Check sheet for the modelled part. Datum: model origin and axes. Units: mm. A direction names the side the tool comes from. Round coordinates to 2 decimals unless told otherwise and drop trailing zeros. Order: outer loops, then holes, each group sorted by start corner. A loop starts at its lowest first (then second) coordinate and runs counter-clockwise, first axis right, second up.
Q1. Cross-section at C-C on z = 2.5. Record the cut outline in (x, y).
Q2. Cross-section at B-B on x = -10. Record the cut outline in (y, z).
Q3. Set-up check for faces 1 (the flat face through (1.905, -122, 20)), 2 (the flat face through (-10.63, -56.35, 6.13)), 3 (the flat face through (0, 5, 19.987)): record each of +Z, -Z, +X, -X, +Y, -Y from which the full face is reachable in a straight line by a thin tool's end or side.
Q4. Scan lines: probe 1 along Z at (x, y) = (-7, -46.5); probe 2 along Z at (x, y) = (-13, -58); probe 3 along Z at (x, y) = (5.5, -43). Record each from-to range of solid material in increasing order.
Q5. Cross-section at A-A on y = -32.5. Record the cut outline in (x, z).
Q6. Depth check by flat-ended pin: P1, Ø6, axis at x = -17.5, z = 14.5, coming from the +Y side; P2, Ø1.1, axis at x = 0.5, y = 6, coming from the +Z side; P3, Ø6, axis at x = -9, z = 11, coming from the -Y side. Enter the tip coordinate at first touch or a pass-through.
Q7. Mould release check, pull along Z, two halves, no side actions. Record for faces 4 (the flat face through (6.61, -56.35, 4.62)), 5 (the flat face through (-1.905, -122, 20)), 6 (the flat face through (0, 6, 23.797)), 7 (the cylindrical face through (17.27, -56.35, 10.71)): +Z half, -Z half, draft (parallel to the pull), parting line (faces both ways), or undercut.
from build123d import *

# Parameters (mm, degrees)
F0_R     = 25.4
F1_DEPTH = 114.3
F2_W     = 3.81
F2_H     = 3.81
F3_DEPTH = 12.7
F4_W     = 3.81
F4_H     = 3.81
F5_DEPTH = 12.7
F6_W     = 3.81
F6_H     = 3.556
F7_DEPTH = 6.35
F8_W     = 3.81
F8_H     = 3.556
F9_DEPTH = 6.35


with BuildPart() as f1:
    # F0 (on Front) → F1 (new body)
    with BuildSketch(Plane.XZ):
        Circle(F0_R)
        with BuildLine():
            ThreePointArc((16.884709, -11.305264), (0.394939, -20.316162), (-16.432577, -11.952941))
            Line((-16.432577, -11.952941), (16.884709, -11.305264))
        make_face(mode=Mode.SUBTRACT)
        with BuildLine():
            ThreePointArc((-18.567839, -8.254559), (-17.791782, 9.816053), (-2.919006, 20.109247))
            Line((-2.919006, 20.109247), (-18.567839, -8.254559))
        make_face(mode=Mode.SUBTRACT)
        Polygon((0.19747, 15.241919), (13.196979, -6.295993), (-11.955155, -6.784942), align=None, mode=Mode.SUBTRACT)
        with BuildLine():
            ThreePointArc((3.221185, 20.06306), (17.396842, 10.500108), (19.252822, -6.498558))
            Line((19.252822, -6.498558), (3.221185, 20.06306))
        make_face(mode=Mode.SUBTRACT)
    extrude(amount=F1_DEPTH)

    # F2 (on face) → F3 (join)
    with BuildSketch(Plane(origin=(0, 0, 0), x_dir=(-1, 0, 0), z_dir=(0, 1, 0))):
        with Locations((0, 21.892242)):
            Rectangle(F2_W, F2_H)
    extrude(amount=F3_DEPTH)

    # F4 (on face) → F5 (join)
    with BuildSketch(Plane.XZ.offset(114.3)):
        with Locations((0, 21.180816)):
            Rectangle(F4_W, F4_H)
    extrude(amount=F5_DEPTH)

    # F6 (on face) → F7 (join)
    with BuildSketch(Plane(origin=(0, 0, 19.987242), x_dir=(1, 0, 0), z_dir=(0, 0, -1))):
        with Locations((0, -10.922)):
            Rectangle(F6_W, F6_H)
    extrude(amount=F7_DEPTH)

    # F8 (on face) → F9 (join)
    with BuildSketch(Plane(origin=(0, 0, 19.275816), x_dir=(1, 0, 0), z_dir=(0, 0, -1))):
        with Locations((0, 125.222)):
            Rectangle(F8_W, F8_H)
    extrude(amount=F9_DEPTH)


solid = f1.part
Results found:
1. outline: (-25.28, -114.3) - (-20.17, -114.3) - (-20.17, 0) - (-25.28, 0) - close; (-12.63, -114.3) - (-6.83, -114.3) - (-6.83, 0) - (-12.63, 0) - close; (7.89, -114.3) - (13.82, -114.3) - (13.82, 0) - (7.89, 0) - close; (20.17, -114.3) - (25.28, -114.3) - (25.28, 0) - (20.17, 0) - close
2. outline: (-114.3, -23.35) - (0, -23.35) - (0, -17.69) - (-114.3, -17.69) - close; (-114.3, -11.83) - (0, -11.83) - (0, -6.75) - (-114.3, -6.75) - close; (-114.3, -3.24) - (0, -3.24) - (0, 7.27) - (-114.3, 7.27) - close; (-114.3, 17.69) - (0, 17.69) - (0, 23.35) - (-114.3, 23.35) - close
3. face 1: +Z, -Z, +X, -Y
3. face 2: +Y, -Y
3. face 3: -Z, +X, -X
4. probe 1: z = -24.42 to -19.08, -11.77 to -6.69, 2.2 to 12.71, 19.08 to 24.42
4. probe 2: z = -21.82 to -15.62, -11.89 to 1.84, 15.62 to 21.82
4. probe 3: z = -24.8 to -19.56, -11.53 to -6.45, 6.46 to 16.29, 19.56 to 24.8
5. outline: circle Ø50.8 at (0, 0); hole (-18.57, -8.25) - (-2.92, 20.11) arc R20.32 ccw to start; hole (-16.43, -11.95) arc R20.32 ccw to (16.88, -11.31) - close; hole (-11.96, -6.78) - (13.2, -6.3) - (0.2, 15.24) - close; hole (3.22, 20.06) - (19.25, -6.5) arc R20.32 ccw to start
6. P1: stops at y = 0
6. P2: stops at z = 23.8
6. P3: stops at y = -114.3
7. face 4: undercut
7. face 5: draft
7. face 6: +Z half
7. face 7: undercut
